Design review of the part built by this model. Coordinates are the model's own, in mm. Face numbers are marked on the shaded views. A direction names the side the tool comes from. Coordinates: 2 decimals unless noted, no trailing zeros. Write each loop counter-clockwise with the first axis right and the second up, starting at its lowest first coordinate (ties: lowest second). Pieces come first, ordered by that corner, then holes.
Q1. For pin 1 Ø2 at (x, z) = (0.5, 10) entering from +Y; pin 2 Ø1.5 at (y, z) = (-1.5, 6.5) entering from +X; pin 3 Ø1 at (x, z) = (-1, 6.5) entering from +Y; pin 4 Ø1.5 at (x, z) = (3, 3) entering from +Y, all flat-tipped, find the tip position at first contact; note any pin that passes through.
Q2. Take a section at A-A, the plane x = 0. Write out the cut boundary in (y, z), plus the area to 3 significant figures.
Q3. Take a section at D-D, the plane x = -2.5. Write out the cut boundary in (y, z), plus the area to 4 significant figures.
Q4. For L1, parallel to Z at x = 0.25, y = -2; L2, parallel to Y at x = 0, z = 8.5; L3, parallel to X at y = 0.25, z = 8, list the stretches that pass through material, from the lowest coordinate up.
Q5. Take a section at C-C, the plane z = 11. Write out the cut boundary in (x, y).
Q6. For the marked faces 1 and 2, list the 3-axis set-ups (+Z, -Z, +X, -X, +Y, -Y) from which the entire face can be reached by the end or side of a thin tool; tool diameter is ignored.
from build123d import *

# Parameters (mm, degrees)
CYLINDER001_R     = 1.97
CYLINDER001_DEPTH = 11.5
CYLINDER_R        = 4
CYLINDER_DEPTH    = 1


with BuildPart() as cylinder001:
    # Cylinder001 → Cylinder001 (new body)
    with BuildSketch(Plane.XY.offset(1)):
        Circle(CYLINDER001_R)
    extrude(amount=CYLINDER001_DEPTH)


with BuildPart() as fusion:
    # Cylinder → Cylinder (new body)
    with BuildSketch(Plane.XY):
        Circle(CYLINDER_R)
    extrude(amount=CYLINDER_DEPTH)

    # Fusion: union Cylinder001
    add(cylinder001.part)


solid = fusion.part
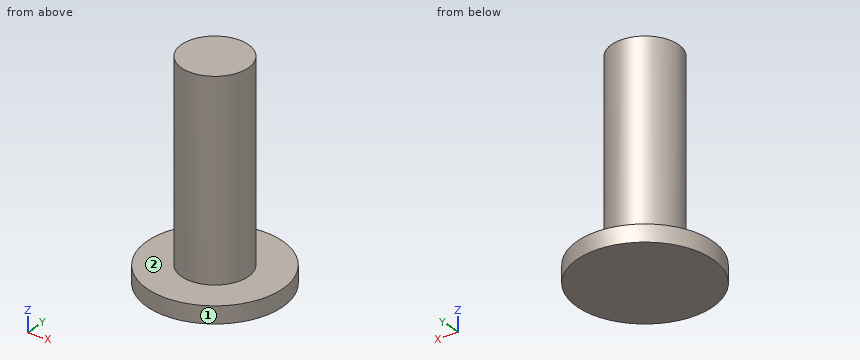
Responses:
1. pin 1: stops at y = 1.97
1. pin 2: stops at x = 1.82
1. pin 3: stops at y = 1.91
1. pin 4: passes through
2. outline: (-4, 0) - (4, 0) - (4, 1) - (1.97, 1) - (1.97, 12.5) - (-1.97, 12.5) - (-1.97, 1) - (-4, 1) - close
2. area: 53.3 mm2
3. outline: (-3.12, 0) - (3.12, 0) - (3.12, 1) - (-3.12, 1) - close
3. area: 6.245 mm2
4. L1: z = 0 to 1
4. L2: y = -1.97 to 1.97
4. L3: x = -1.95 to 1.95
5. outline: circle Ø3.94 at (0, 0)
6. face 1: +Z, -Z
6. face 2: +Z
